Build history of the part. All positions in model axes, mm. Face numbers are marked on the shaded views. A direction names the side the tool comes from. Coordinates: 2 decimals unless noted, no trailing zeros. Write each loop counter-clockwise with the first axis right and the second up, starting at its lowest first coordinate (ties: lowest second). Pieces come first, ordered by that corner, then holes. Notation, with made-up numbers: (-26.5, -12.5) -> (-15.5, -12.5) arc R12 ccw to (-15.5, 3.5) -> close; hole circle Ø4 at (-5, 67.5). An arc over 180 degrees is marked (long way). Write each question's results on one line, items separated by ' | '. Start each with the question number.
Q1. Two-plate mould, pull along X, no slides. Class the marked faces 4, 5 and 6: released by +X, released by -X, zero draft, split by the parting line, or undercut.
Q2. Drop flat-ended pins along their axis: pin 1 Ø4 at (x, z) = (-0.5, 0.5) entering from +Y; pin 2 Ø12 at (x, y) = (3.5, 2) entering from -Z; pin 3 Ø1.5 at (y, z) = (-2, -0.5) entering from +X; pin 4 Ø1 at (x, z) = (-4, 4) entering from +Y. Give the stop position or say it passes through.
Q3. Saw through at C-C on z = -4.75. Give the cut face in (x, y).
Q4. Saw through at D-D on z = -1. Give the cut face in (x, y), and give its area (3 significant figures).
Q5. Saw through at B-B on x = -8. Give the cut face in (y, z).
Q6. Tool access for the marked faces 1, 2 and 3: list every direction of +Z, -Z, +X, -X, +Y, -Y with a clear straight run to the whole face (end or side of a thin tool).
Q7. Drill centre lines: line 1 (Y direction, x = 0, z = -6.75); line 2 (Z direction, x = 16.5, y = -4); line 3 (X direction, y = -15.5, z = 1.75). Where is each one in solid material? Low to high.
Q8. Saw through at A-A on y = 1. Give the cut face in (x, z), and give its area (3 significant figures).
from build123d import *

# Parameters (mm, degrees)
BOSS_EXTRUDE1_DEPTH = 5
SKETCH2_R           = 20
BOSS_EXTRUDE2_DEPTH = 1.5
BOSS_EXTRUDE3_START = 1.5
SKETCH3_R           = 20
BOSS_EXTRUDE3_DEPTH = 1.5
SKETCH4_R           = 13
CUT_EXTRUDE1_DEPTH  = 11.5
SKETCH5_R           = 15
BOSS_EXTRUDE4_DEPTH = 10
CUT_EXTRUDE2_START  = -30
SKETCH6_R           = 13
CUT_EXTRUDE2_DEPTH  = 30


with BuildPart() as part:
    # Sketch1 → Boss-Extrude1 (new body)
    with BuildSketch(Plane.XY):
        with BuildLine():
            Line((0, 17), (-1.990617103, 13.857757522))
            ThreePointArc((-1.990617103, 13.857757522), (-2.190082511, 13.827636768), (-2.389093211, 13.794645107))
            Line((-2.389093211, 13.794645107), (-5.253288904, 16.167960777))
            Line((-5.253288904, 16.167960777), (-6.175471945, 12.564376079))
            ThreePointArc((-6.175471945, 12.564376079), (-6.355866996, 12.474091339), (-6.534942436, 12.381216715))
            Line((-6.534942436, 12.381216715), (-9.992349289, 13.753288904))
            Line((-9.992349289, 13.753288904), (-9.755828567, 10.041105964))
            ThreePointArc((-9.755828567, 10.041105964), (-9.899494937, 9.899494937), (-10.041105964, 9.755828567))
            Line((-10.041105964, 9.755828567), (-13.753288904, 9.992349289))
            Line((-13.753288904, 9.992349289), (-12.381216715, 6.534942436))
            ThreePointArc((-12.381216715, 6.534942436), (-12.474091339, 6.355866996), (-12.564376079, 6.175471945))
            Line((-12.564376079, 6.175471945), (-16.167960777, 5.253288904))
            Line((-16.167960777, 5.253288904), (-13.794645107, 2.389093211))
            ThreePointArc((-13.794645107, 2.389093211), (-13.827636768, 2.190082511), (-13.857757522, 1.990617103))
            Line((-13.857757522, 1.990617103), (-17, 0))
            Line((-17, 0), (-13.857757522, -1.990617103))
            ThreePointArc((-13.857757522, -1.990617103), (-13.827636768, -2.190082511), (-13.794645107, -2.389093211))
            Line((-13.794645107, -2.389093211), (-16.167960777, -5.253288904))
            Line((-16.167960777, -5.253288904), (-12.564376079, -6.175471945))
            ThreePointArc((-12.564376079, -6.175471945), (-12.474091339, -6.355866996), (-12.381216715, -6.534942436))
            Line((-12.381216715, -6.534942436), (-13.753288904, -9.992349289))
            Line((-13.753288904, -9.992349289), (-10.041105964, -9.755828567))
            ThreePointArc((-10.041105964, -9.755828567), (-9.899494937, -9.899494937), (-9.755828567, -10.041105964))
            Line((-9.755828567, -10.041105964), (-9.992349289, -13.753288904))
            Line((-9.992349289, -13.753288904), (-6.534942436, -12.381216715))
            ThreePointArc((-6.534942436, -12.381216715), (-6.355866996, -12.474091339), (-6.175471945, -12.564376079))
            Line((-6.175471945, -12.564376079), (-5.253288904, -16.167960777))
            Line((-5.253288904, -16.167960777), (-2.389093211, -13.794645107))
            ThreePointArc((-2.389093211, -13.794645107), (-2.190082511, -13.827636768), (-1.990617103, -13.857757522))
            Line((-1.990617103, -13.857757522), (0, -17))
            Line((0, -17), (1.990617103, -13.857757522))
            ThreePointArc((1.990617103, -13.857757522), (2.190082511, -13.827636768), (2.389093211, -13.794645107))
            Line((2.389093211, -13.794645107), (5.253288904, -16.167960777))
            Line((5.253288904, -16.167960777), (6.175471945, -12.564376079))
            ThreePointArc((6.175471945, -12.564376079), (6.355866996, -12.474091339), (6.534942436, -12.381216715))
            Line((6.534942436, -12.381216715), (9.992349289, -13.753288904))
            Line((9.992349289, -13.753288904), (9.755828567, -10.041105964))
            ThreePointArc((9.755828567, -10.041105964), (9.899494937, -9.899494937), (10.041105964, -9.755828567))
            Line((10.041105964, -9.755828567), (13.753288904, -9.992349289))
            Line((13.753288904, -9.992349289), (12.381216715, -6.534942436))
            ThreePointArc((12.381216715, -6.534942436), (12.474091339, -6.355866996), (12.564376079, -6.175471945))
            Line((12.564376079, -6.175471945), (16.167960777, -5.253288904))
            Line((16.167960777, -5.253288904), (13.794645107, -2.389093211))
            ThreePointArc((13.794645107, -2.389093211), (13.827636768, -2.190082511), (13.857757522, -1.990617103))
            Line((13.857757522, -1.990617103), (17, 0))
            Line((17, 0), (13.857757522, 1.990617103))
            ThreePointArc((13.857757522, 1.990617103), (13.827636768, 2.190082511), (13.794645107, 2.389093211))
            Line((13.794645107, 2.389093211), (16.167960777, 5.253288904))
            Line((16.167960777, 5.253288904), (12.564376079, 6.175471945))
            ThreePointArc((12.564376079, 6.175471945), (12.474091339, 6.355866996), (12.381216715, 6.534942436))
            Line((12.381216715, 6.534942436), (13.753288904, 9.992349289))
            Line((13.753288904, 9.992349289), (10.041105964, 9.755828567))
            ThreePointArc((10.041105964, 9.755828567), (9.899494937, 9.899494937), (9.755828567, 10.041105964))
            Line((9.755828567, 10.041105964), (9.992349289, 13.753288904))
            Line((9.992349289, 13.753288904), (6.534942436, 12.381216715))
            ThreePointArc((6.534942436, 12.381216715), (6.355866996, 12.474091339), (6.175471945, 12.564376079))
            Line((6.175471945, 12.564376079), (5.253288904, 16.167960777))
            Line((5.253288904, 16.167960777), (2.389093211, 13.794645107))
            ThreePointArc((2.389093211, 13.794645107), (2.190082511, 13.827636768), (1.990617103, 13.857757522))
            Line((1.990617103, 13.857757522), (0, 17))
        make_face()
    extrude(amount=BOSS_EXTRUDE1_DEPTH)

    # Sketch2 → Boss-Extrude2 (add)
    with BuildSketch(Plane(origin=(0, 0, 0), x_dir=(-1, 0, 0), z_dir=(0, 0, -1))):
        Circle(SKETCH2_R)
    extrude(amount=BOSS_EXTRUDE2_DEPTH)

    # Sketch3 → Boss-Extrude3 (add)
    with BuildSketch(Plane.XY.offset(5).offset(BOSS_EXTRUDE3_START)):
        with Locations(Location((0, 0, 0), (0, 0, 180))):
            Circle(SKETCH3_R)
    extrude(amount=-BOSS_EXTRUDE3_DEPTH)

    # Sketch4 → Cut-Extrude1 (cut)
    with BuildSketch(Plane.XY.offset(6.5)):
        Circle(SKETCH4_R)
    extrude(amount=-CUT_EXTRUDE1_DEPTH, mode=Mode.SUBTRACT)

    # Sketch5 → Boss-Extrude4 (add)
    with BuildSketch(Plane(origin=(0, 0, -1.5), x_dir=(-1, 0, 0), z_dir=(0, 0, -1))):
        Circle(SKETCH5_R)
    extrude(amount=BOSS_EXTRUDE4_DEPTH)

    # Sketch6 → Cut-Extrude2 (cut)
    with BuildSketch(Plane(origin=(0, 0, -11.5), x_dir=(-1, 0, 0), z_dir=(0, 0, -1)).offset(CUT_EXTRUDE2_START)):
        with Locations(Location((0, 0, 0), (0, 0, 180))):
            Circle(SKETCH6_R)
    extrude(amount=CUT_EXTRUDE2_DEPTH, mode=Mode.SUBTRACT)


solid = part.part
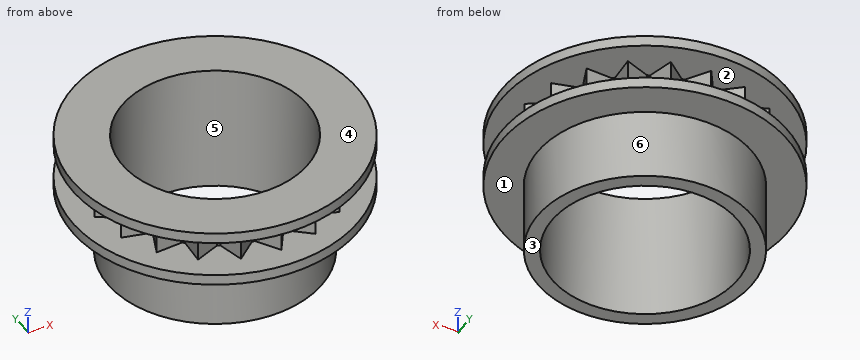
Returned:
1) face 4: zero draft | face 5: undercut | face 6: split by the parting line
2) pin 1: stops at y = 20 | pin 2: passes through | pin 3: stops at x = 19.96 | pin 4: stops at y = 15.54
3) outline: circle Ø30 at (0, 0); hole circle Ø26 at (0, 0)
4) outline: circle Ø40 at (0, 0); hole circle Ø26 at (0, 0) | area: 726 mm2
5) outline: (-18.33, -1.5) -> (-12.69, -1.5) -> (-12.69, -11.5) -> (-10.25, -11.5) -> (-10.25, 6.5) -> (-18.33, 6.5) -> (-18.33, 5) -> (-12.96, 5) -> (-12.96, 0) -> (-18.33, 0) -> close; (10.25, -11.5) -> (12.69, -11.5) -> (12.69, -1.5) -> (18.33, -1.5) -> (18.33, 0) -> (12.96, 0) -> (12.96, 5) -> (18.33, 5) -> (18.33, 6.5) -> (10.25, 6.5) -> close
6) face 1: -Z | face 2: none | face 3: -Z, +X, -X, +Y, -Y
7) line 1: y = -15 to -13, 13 to 15 | line 2: z = -1.5 to 0, 5 to 6.5 | line 3: x = -5.42 to -4.45, -0.95 to 0.95, 4.45 to 5.42
8) outline: (-19.97, -1.5) -> (-14.97, -1.5) -> (-14.97, -11.5) -> (-12.96, -11.5) -> (-12.96, 6.5) -> (-19.97, 6.5) -> (-19.97, 5) -> (-15.42, 5) -> (-15.42, 0) -> (-19.97, 0) -> close; (12.96, -11.5) -> (14.97, -11.5) -> (14.97, -1.5) -> (19.97, -1.5) -> (19.97, 0) -> (15.42, 0) -> (15.42, 5) -> (19.97, 5) -> (19.97, 6.5) -> (12.96, 6.5) -> close | area: 107 mm2
